Autodesk Inventor part; units mm, degrees
ref_plane "YZ Plane" through (0, 0, 0) normal (1, 0, 0) x (0, 1, 0)
ref_plane "XZ Plane" through (0, 0, 0) normal (0, 1, 0) x (-1, 0, 0)
ref_plane "XY Plane" through (0, 0, 0) normal (0, 0, 1) x (1, 0, 0)
sketch "Sketch1" plane through (0, 0, 0) normal (0, 1, 0) x (-1, 0, 0)
  circle A0 centre (0, 0) radius 21.5
  circle A1 centre (0, -18) radius 1.5
  circle A2 centre (15.5885, -9) radius 1.5
  circle A3 centre (15.5885, 9) radius 1.5
  circle A4 centre (0, 18) radius 1.5
  circle A5 centre (-15.5885, 9) radius 1.5
  circle A6 centre (-15.5885, -9) radius 1.5
  dimension "d0" = 43
  dimension "d1" = 3
  dimension "d2" = 18
  dimension "d5" = 360
extrude "Extrusion1" add sketch "Sketch1" along normal blind 4
sketch "Sketch2" plane through (0, 4, 0) normal (0, 1, 0) x (1, 0, 0)
  circle A0 centre (0, 0) radius 16
  dimension "d9" = 32
extrude "Extrusion2" add sketch "Sketch2" along normal blind 4
sketch "Sketch3" plane through (0, 8, 0) normal (0, 1, 0) x (1, 0, 0)
  circle A0 centre (0, 12) radius 2.1
  circle A1 centre (-8.4853, 8.4853) radius 2.1
  circle A2 centre (-12, 0) radius 2.1
  circle A3 centre (-8.4853, -8.4853) radius 2.1
  circle A4 centre (0, -12) radius 2.1
  circle A5 centre (8.4853, -8.4853) radius 2.1
  circle A6 centre (12, 0) radius 2.1
  circle A7 centre (8.4853, 8.4853) radius 2.1
  point P0 (0, 0)
  dimension "d27" = 4.2
  dimension "d32" = 360
  dimension "d44" = 12
extrude "Extrusion3" cut sketch "Sketch3" against normal blind 4
thread "Thread7"
thread "Thread8"
thread "Thread9"
thread "Thread10"
thread "Thread11"
thread "Thread12"
thread "Thread13"
thread "Thread14"
thread "Thread15"
thread "Thread16"
thread "Thread17"
thread "Thread18"
thread "Thread19"
thread "Thread20"
sketch "Sketch4" plane through (0, 0, 0) normal (0, -1, 0) x (1, 0, 0)
  circle A0 centre (0, 0) radius 6
  dimension "d65" = 12
extrude "Extrusion4" cut sketch "Sketch4" against normal blind 5
properties part number "OutPutPlate" material "Aluminum 6061"
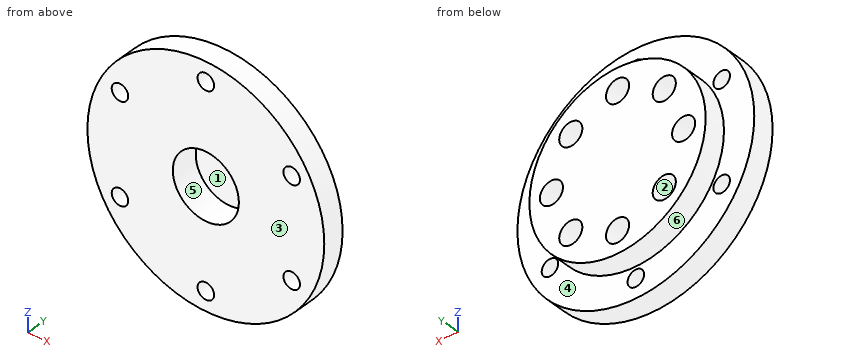
Could you check a few things on this model? Use its own coordinates, in mm. Face numbers are marked on the shaded views. A direction names the side the tool comes from. Round coordinates to 2 decimals unless told otherwise and drop trailing zeros. Order: outer loops, then holes, each group sorted by start corner. A loop starts at its lowest first (then second) coordinate and runs counter-clockwise, first axis right, second up.
Q1. Please list where these lines run through material, in increasing order: probe 1 along Z at (x, y) = (0, 0.85); probe 2 along Z at (x, y) = (-14.5, 3); probe 3 along Z at (x, y) = (16, 3.75).
Geometry says:
probe 1: z = -21.5 to -19.5, -16.5 to -6, 6 to 16.5, 19.5 to 21.5
probe 2: z = -15.87 to -10.03, -7.97 to 7.97, 10.03 to 15.87
probe 3: z = -14.36 to -10.44, -7.56 to 7.56, 10.44 to 14.36
Q2. Imagine slicing it at A-A, the plane x = 0. List the corners of the cut face in (y, z) for me.
Geometry says:
outline: (0, -21.5) - (4, -21.5) - (4, -19.5) - (0, -19.5) - close; (0, -16.5) - (4, -16.5) - (4, -16) - (8, -16) - (8, -14.1) - (4, -14.1) - (4, -9.9) - (8, -9.9) - (8, 9.9) - (4, 9.9) - (4, 14.1) - (8, 14.1) - (8, 16) - (4, 16) - (4, 16.5) - (0, 16.5) - (0, 6) - (5, 6) - (5, -6) - (0, -6) - close; (0, 19.5) - (4, 19.5) - (4, 21.5) - (0, 21.5) - close
Q3. I'm going to push flat-ended pins straight in: P1, Ø1.3, axis at x = 9, z = 7.5, coming from the +Y side; P2, Ø3, axis at y = 2, z = 15.5, coming from the -X side; P3, Ø1.5, axis at x = 8.5, y = 4.5, coming from the -Z side. Where does each tip first touch, or does it pass through?
Geometry says:
P1: stops at y = 4
P2: stops at x = -16.32
P3: stops at z = -19.98
Q4. Which directions (+Z, -Z, +X, -X, +Y, -Y) give clear straight access to the entire face, cutting with the end or side of a thin tool? Please do the marked faces 1, 2 and 3.
Geometry says:
face 1: -Y
face 2: +Y
face 3: +Z, -Z, +X, -X, -Y
Q5. Imagine slicing it at D-D, the plane y = 6.5. State how many separate pieces and enclosed holes the cut face has, then the cut area to 3 significant figures.
Geometry says:
separate pieces: 1
enclosed holes: 8
area: 693 mm2
Q6. Thinking about a two-plate mould opening in X: for the marked faces 4, 5 and 6, which applies, released by +X, released by -X, zero draft, split by the parting line, or undercut?
Geometry says:
face 4: zero draft
face 5: undercut
face 6: split by the parting line
Q7. Imagine slicing it at C-C, the plane y = 0.5. List the corners of the cut face in (x, z) for me.
Geometry says:
outline: circle Ø43 at (0, 0); hole circle Ø3 at (-15.59, -9); hole circle Ø3 at (-15.59, 9); hole circle Ø12 at (0, 0); hole circle Ø3 at (0, -18); hole circle Ø3 at (0, 18); hole circle Ø3 at (15.59, -9); hole circle Ø3 at (15.59, 9)
Q8. Imagine slicing it at B-B, the plane z = 9. List the corners of the cut face in (x, y) for me.
Geometry says:
outline: (-19.53, 0) - (-17.09, 0) - (-17.09, 4) - (-19.53, 4) - close; (-14.09, 0) - (14.09, 0) - (14.09, 4) - (13.23, 4) - (13.23, 8) - (10.52, 8) - (10.52, 4) - (6.45, 4) - (6.45, 8) - (-6.45, 8) - (-6.45, 4) - (-10.52, 4) - (-10.52, 8) - (-13.23, 8) - (-13.23, 4) - (-14.09, 4) - close; (17.09, 0) - (19.53, 0) - (19.53, 4) - (17.09, 4) - close
